Input: part model. Units: mm. Frame: model coordinates. Face numbers are marked on the shaded views. Give positions to 0.01 mm unless a question says otherwise; leave off trailing zeros. Loops run counter-clockwise (first coordinate to the right, second up) from the corner with the lowest first, then second, coordinate; pieces in that order, holes last. Notation, with made-up numbers: (6, -17) -> (17, -17) arc R27 ccw to (17, 21) -> close; hole circle Ø11 at (-21.5, -13). An arc over 180 degrees is marked (long way). Use CSV: the item, a comma, the result in double quotes.
Autodesk Inventor part; units mm, degrees
ref_plane "YZ Plane" through (0, 0, 0) normal (1, 0, 0) x (0, 1, 0)
ref_plane "XZ Plane" through (0, 0, 0) normal (0, 1, 0) x (-1, 0, 0)
ref_plane "XY Plane" through (0, 0, 0) normal (0, 0, 1) x (1, 0, 0)
sketch "Sketch1" plane through (0, 0, 0) normal (0, 0, 1) x (1, 0, 0)
  line L0 (0, 81.9) -> (0, -81.9)
  line L1 (-56, 0) -> (56, 0)
  line L2 (-40, 58.5) -> (40, 58.5)
  line L3 (40, 58.5) -> (40, -58.5)
  line L4 (40, -58.5) -> (-40, -58.5)
  line L5 (-40, -58.5) -> (-40, 58.5)
  point P0 (0, 0)
  dimension "d0" = 80
  dimension "d1" = 117
extrude "Extrusion1" add sketch "Sketch1" along normal blind 8
sketch "Sketch2" plane through (0, 0, 8) normal (0, 0, 1) x (1, 0, 0)
  line L0 (40, 58.5) -> (-40, 58.5)
  line L1 (-40, 58.5) -> (-40, -58.5)
  line L2 (-40, -58.5) -> (40, -58.5)
  line L3 (40, -58.5) -> (40, 58.5)
  line L4 (-56, 0) -> (56, 0)
  line L5 (0, -81.9) -> (0, 81.9)
  line L6 (-32, 0) -> (-1.8784, 0)
  line L7 (-1.8784, 0) -> (-1.8784, -3)
  line L8 (-1.8784, -3) -> (-32, -3)
  line L9 (-32, -3) -> (-32, 0)
  line L10 (-25, -15) -> (-25, -20)
  line L11 (-25, -20) -> (-30, -20)
  line L12 (-30, -20) -> (-30, -25)
  line L13 (-30, -25) -> (-25, -25)
  line L14 (-25, -25) -> (-25, -30)
  line L15 (-25, -30) -> (-20, -30)
  line L16 (-20, -30) -> (-20, -25)
  line L17 (-20, -25) -> (-15, -25)
  line L18 (-15, -25) -> (-15, -20)
  line L19 (-15, -20) -> (-20, -20)
  line L20 (-20, -20) -> (-20, -15)
  line L21 (-20, -15) -> (-25, -15)
  line L22 (14, -14) -> (10, -20.9282)
  line L23 (10, -20.9282) -> (18, -20.9282)
  circle A0 centre (27, -22) radius 3
  circle A1 centre (18, -32) radius 5
  line L24 (-32, -42) -> (-22, -42)
  line L25 (-22, -42) -> (-22, -45.5)
  line L26 (-22, -45.5) -> (-32, -45.5)
  line L27 (-32, -45.5) -> (-32, -42)
  line L28 (-14, -42) -> (-4, -42)
  line L29 (-4, -42) -> (-4, -45.5)
  line L30 (-4, -45.5) -> (-14, -45.5)
  line L31 (-14, -45.5) -> (-14, -42)
  circle A2 centre (30.5, -1.5) radius 1.5
  line L32 (14, -20.9282) -> (14, -9.9927) construction
  line L33 (14, -14) -> (18, -20.9282)
  line L34 (-1.8784, -1.5) -> (30.5, -1.5) construction
  line L35 (-32, 50.5) -> (32, 50.5) construction
  line L36 (32, 50.5) -> (32, 8) construction
  line L37 (32, 8) -> (-32, 8) construction
  line L38 (-32, 8) -> (-32, 50.5) construction
  point P0 (0, 0)
  dimension "d4" = 3
  dimension "d5" = 8
  dimension "d7" = 5
  dimension "d8" = 60
  dimension "d9" = 10
  dimension "d10" = 12
  dimension "d11" = 12
  dimension "d12" = 3
  dimension "d13" = 8
  dimension "d14" = 8
  dimension "d15" = 8
  dimension "d16" = 10
  dimension "d17" = 22
  dimension "d18" = 22
  dimension "d19" = 22
  dimension "d20" = 40
  dimension "d21" = 30
  dimension "d22" = 13
  dimension "d23" = 6
  dimension "d24" = 10
  dimension "d25" = 13
  dimension "d26" = 8
extrude "Extrusion2" add sketch "Sketch2" along normal blind 2 contours A2 | L7 L8 L9 L4 | L21 L20 L19 L18 L17 L16 L15 L14 L13 L12 L11 L10 | L33 L23 L22 | A0 | A1 | L24 L25 L26 L27 | L28 L29 L30 L31
sketch "Sketch3" plane through (0, 0, 8) normal (0, 0, 1) x (1, 0, 0)
  line L0 (-32, 0) -> (-1.8784, 0)
  line L1 (-1.8784, 0) -> (-1.8784, -3)
  line L2 (-1.8784, -3) -> (-32, -3)
  line L3 (-32, -3) -> (-32, 0)
  line L4 (-4, -42) -> (-4, -45.5)
  line L5 (-4, -45.5) -> (-14, -45.5)
  line L6 (-14, -45.5) -> (-14, -42)
  line L7 (-14, -42) -> (-4, -42)
  circle A0 centre (27, -22) radius 3
  circle A1 centre (30.5, -1.5) radius 1.5
  line L8 (14, -14) -> (18, -20.9282)
  line L9 (18, -20.9282) -> (10, -20.9282)
  line L10 (10, -20.9282) -> (14, -14)
  line L11 (-22, -42) -> (-22, -45.5)
  line L12 (-22, -45.5) -> (-32, -45.5)
  line L13 (-32, -45.5) -> (-32, -42)
  line L14 (-32, -42) -> (-22, -42)
  circle A2 centre (18, -32) radius 5
  line L15 (-25, -15) -> (-20, -15)
  line L16 (-20, -15) -> (-20, -20)
  line L17 (-20, -20) -> (-15, -20)
  line L18 (-15, -20) -> (-15, -25)
  line L19 (-15, -25) -> (-20, -25)
  line L20 (-20, -25) -> (-20, -30)
  line L21 (-20, -30) -> (-25, -30)
  line L22 (-25, -30) -> (-25, -25)
  line L23 (-25, -25) -> (-30, -25)
  line L24 (-30, -25) -> (-30, -20)
  line L25 (-30, -20) -> (-25, -20)
  line L26 (-25, -20) -> (-25, -15)
  line L27 (40, 58.5) -> (-40, 58.5)
  line L28 (-40, 58.5) -> (-40, -58.5)
  line L29 (-40, -58.5) -> (40, -58.5)
  line L30 (40, -58.5) -> (40, 58.5)
  line L31 (-32, 50.5) -> (32, 50.5)
  line L32 (32, 50.5) -> (32, 8)
  line L33 (32, 8) -> (-32, 8)
  line L34 (-32, 8) -> (-32, 50.5)
  line L35 (-56, 0) -> (56, 0)
  line L36 (0, -81.9) -> (0, 81.9)
  point P0 (0, 0)
  dimension "d29" = 8
  dimension "d30" = 8
  dimension "d31" = 8
extrude "Extrusion3" cut sketch "Sketch3" against normal blind 2 contours L36 L31 L32 L33 | L33 L34 L31 L36
sketch "Sketch4" plane through (0, 0, 6) normal (0, 0, 1) x (1, 0, 0)
  line L0 (-32, 50.5) -> (32, 50.5)
  line L1 (-32, 8) -> (-32, 50.5)
  line L2 (32, 8) -> (-32, 8)
  line L3 (32, 50.5) -> (32, 8)
  line L4 (32, 50.5) -> (32, 8)
  arc A0 (-16.4483, 24.1223) -> (16.4483, 24.1223) centre (0, 35.5) ccw
  arc A1 (-17.9287, 23.0983) -> (17.9287, 23.0983) centre (0, 35.5) ccw
  line L5 (-17.9287, 23.0983) -> (-16.4483, 24.1223)
  line L6 (16.4483, 24.1223) -> (17.9287, 23.0983)
  line L7 (-56, 0) -> (56, 0)
  line L8 (0, -81.9) -> (0, 81.9)
  circle A2 centre (-19, 37.5) radius 4
  circle A3 centre (19, 37.5) radius 4
  point P0 (0, 0)
  dimension "d36" = 1.8
  dimension "d41" = 20
  dimension "d42" = 15
  dimension "d43" = 1.024
  dimension "d44" = 8
  dimension "d45" = 13
  dimension "d46" = 13
extrude "Extrusion6" add sketch "Sketch4" along normal blind 2 contours L8 A1 L5 A0 | A0 L6 A1 L8 | A2 | A3
fillet "Fillet1" [suppressed]
sketch "Sketch5" plane through (0, 0, 0) normal (0, 0, -1) x (-1, 0, 0)
  line L0 (40, 58.5) -> (-40, 58.5)
  line L1 (-40, 58.5) -> (-40, -58.5)
  line L2 (-40, -58.5) -> (40, -58.5)
  line L3 (40, -58.5) -> (40, 58.5)
  circle A0 centre (-35, 53.5) radius 2.75
  line L4 (56, 0) -> (-56, 0)
  line L5 (0, -81.9) -> (0, 81.9)
  circle A1 centre (35, 53.5) radius 2.75
  circle A2 centre (-35, -53.5) radius 2.75
  circle A3 centre (35, -53.5) radius 2.75
  point P0 (0, 0)
  dimension "d51" = 5.5
  dimension "d52" = 5
  dimension "d53" = 5
extrude "Extrusion7" cut sketch "Sketch5" against normal blind 4 contours A0 | A1 | A2 | A3
fillet "Fillet2" radius 2 8 edges at (0, 58.5, 8) (40, 58.5, 4) (40, 0, 8) (-40, 58.5, 4) (-40, 0, 8) (40, -58.5, 4) (0, -58.5, 8) (-40, -58.5, 4)
fillet "Fillet3" radius 0.8 4 edges at (37.75, -53.5, 0) (-32.25, -53.5, 0) (37.75, 53.5, 0) (-32.25, 53.5, 0)
equation "\"d12\" = d4"
equation "\"d14\" = d13"
properties part number "cara"
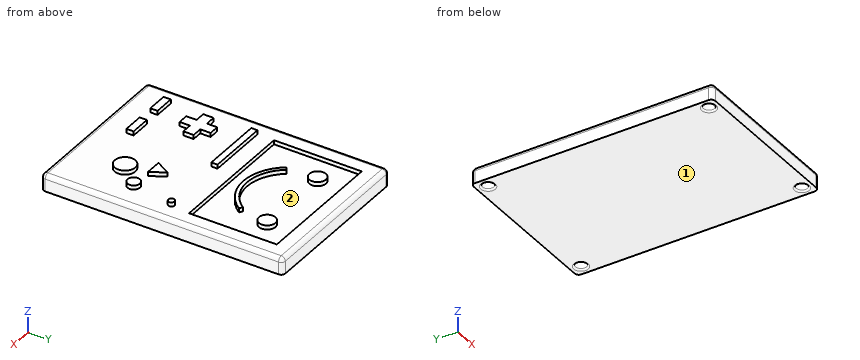
1) Section query C-C (y = -32). Return loops of the section in (x, z).
From the geometry:
outline,"(-40, 0) -> (40, 0) -> (40, 6) arc R2 ccw to (38, 8) -> (23, 8) -> (23, 10) -> (13, 10) -> (13, 8) -> (-38, 8) arc R2 ccw to (-40, 6) -> close"
2) Ray query, line 1 (Y direction, x = -35, z = 1.85); line 2 (Y direction, x = 37.5, z = 2); line 3 (Z direction, x = -16, y = 7.5). Return the intervals inside material, ascending.
From the geometry:
line 1,"y = -58.5 to -56.25, -50.75 to 50.75, 56.25 to 58.5"
line 2,"y = -58.5 to -54.65, -52.35 to 52.35, 54.65 to 58.5"
line 3,"z = 0 to 8"
3) Section query B-B (x = 27). Return loops of the section in (y, z), then the cut area to 3 significant figures.
From the geometry:
outline,"(-58.5, 0) -> (58.5, 0) -> (58.5, 6) arc R2 ccw to (56.5, 8) -> (50.5, 8) -> (50.5, 6) -> (8, 6) -> (8, 8) -> (-19, 8) -> (-19, 10) -> (-25, 10) -> (-25, 8) -> (-56.5, 8) arc R2 ccw to (-58.5, 6) -> close"
area,"861 mm^2"
4) Contact query for flat-ended pins moving along their axis: pin 1 (4 mm diameter, centred on x = -18, y = 35.5, fed in from +Z); pin 2 (0.6 mm diameter, centred on x = -26, z = 9, fed in from +Y); pin 3 (0.6 mm diameter, centred on y = -18.5, z = 8.5, fed in from -X). Output: stop coordinate, or through.
From the geometry:
pin 1,"stops at z = 8"
pin 2,"stops at y = 0"
pin 3,"stops at x = -25"
5) Section query A-A (y = 47). Return loops of the section in (x, z).
From the geometry:
outline,"(-40, 0) -> (40, 0) -> (40, 6) arc R2 ccw to (38, 8) -> (32, 8) -> (32, 6) -> (-32, 6) -> (-32, 8) -> (-38, 8) arc R2 ccw to (-40, 6) -> close"
6) Mould query, pull axis Y, two halves, no side actions, for the marked faces 1 and 2. Classes: pulls with the +Y half, pulls with the -Y half, needs draft (parallel to the pull), parting line crosses it, or undercut.
From the geometry:
face 1,"needs draft"
face 2,"undercut"
7) Section query D-D (x = -35). Return loops of the section in (y, z).
From the geometry:
outline,"(-58.5, 0) -> (-57.05, 0) arc R0.8 ccw to (-56.25, 0.8) -> (-56.25, 4) -> (-50.75, 4) -> (-50.75, 0.8) arc R0.8 ccw to (-49.95, 0) -> (49.95, 0) arc R0.8 ccw to (50.75, 0.8) -> (50.75, 4) -> (56.25, 4) -> (56.25, 0.8) arc R0.8 ccw to (57.05, 0) -> (58.5, 0) -> (58.5, 6) arc R2 ccw to (56.5, 8) -> (-56.5, 8) arc R2 ccw to (-58.5, 6) -> close"
